```python
from build123d import *

# Parameters (mm, degrees)
BOSS_EXTRUDE1_DEPTH       = 35
BOSS_EXTRUDE3_DEPTH       = 1.5
SKETCH5_W                 = 1
SKETCH5_H                 = 1
BOSS_EXTRUDE4_DEPTH       = 18.1
CUT_EXTRUDE2_DEPTH        = 18.1
SKETCH9_W                 = 1
SKETCH9_H                 = 0.5
BOSS_EXTRUDE5_DEPTH       = 0.5
CUT_EXTRUDE3_REACH        = 41.512
SKETCH10_R                = 0.125
SKETCH11_R                = 2.5
BOSS_EXTRUDE6_DEPTH       = 1.5
SKETCH23_R                = 0.5
CUT_EXTRUDE12_DEPTH       = 1.5
SKETCH26_W                = 6.749879612
SKETCH26_H                = 8.598416767
SKETCH26_W_2              = 5.749879612
SKETCH26_H_2              = 7.598416767
BOSS_EXTRUDE16_DEPTH      = 2.05
BOSS_EXTRUDE23_REACH      = 41.419
BOSS_EXTRUDE23_END_RADIUS = 2.5
SKETCH27_W                = 0.594319842
SKETCH27_H                = 0.457567035
SKETCH27_R                = 0.154135996
SKETCH28_W                = 6.749879612
SKETCH28_H                = 8.598416767
BOSS_EXTRUDE24_DEPTH      = 0.5
SKETCH29_R                = 0.154135996
CUT_EXTRUDE13_DEPTH       = 2.5
SKETCH30_R                = 1.735676045
CUT_EXTRUDE14_DEPTH       = 0.5


with BuildPart() as part:
    # Sketch1 → Boss-Extrude1 (new body)
    with BuildSketch(Plane.XY):
        with BuildLine():
            Line((10.3, 6.55), (10.3, -6.55))
            ThreePointArc((10.3, -6.55), (9.567766953, -8.317766953), (7.8, -9.05))
            Line((7.8, -9.05), (-7.8, -9.05))
            Line((-7.8, -9.05), (-7.8, 9.05))
            Line((-7.8, 9.05), (7.8, 9.05))
            ThreePointArc((7.8, 9.05), (9.567766953, 8.317766953), (10.3, 6.55))
        make_face()
        with BuildLine():
            Line((-6.3, 7.55), (7.8, 7.55))
            ThreePointArc((7.8, 7.55), (8.507106781, 7.257106781), (8.8, 6.55))
            Line((8.8, 6.55), (8.8, -6.55))
            ThreePointArc((8.8, -6.55), (8.507106781, -7.257106781), (7.8, -7.55))
            Line((7.8, -7.55), (-6.3, -7.55))
            Line((-6.3, -7.55), (-6.3, 7.55))
        make_face(mode=Mode.SUBTRACT)
    extrude(amount=BOSS_EXTRUDE1_DEPTH)

    # Sketch4 → Boss-Extrude3 (add)
    with BuildSketch(Plane(origin=(0, 0, 0), x_dir=(-1, 0, 0), z_dir=(0, 0, -1))):
        with BuildLine():
            Line((7.8, -9.05), (7.8, 9.05))
            Line((7.8, 9.05), (-7.8, 9.05))
            ThreePointArc((-7.8, 9.05), (-9.567766953, 8.317766953), (-10.3, 6.55))
            Line((-10.3, 6.55), (-10.3, -6.55))
            ThreePointArc((-10.3, -6.55), (-9.567766953, -8.317766953), (-7.8, -9.05))
            Line((-7.8, -9.05), (7.8, -9.05))
        make_face()
    extrude(amount=-BOSS_EXTRUDE3_DEPTH)

    # Sketch5 → Boss-Extrude4 (add)
    with BuildSketch(Plane.XZ.offset(9.05)):
        with Locations((-8.3, 15)):
            Rectangle(SKETCH5_W, SKETCH5_H)
        with Locations((-8.3, 30)):
            Rectangle(SKETCH5_W, SKETCH5_H)
    extrude(amount=-BOSS_EXTRUDE4_DEPTH)

    # Sketch8 → Cut-Extrude2 (cut)
    with BuildSketch(Plane.ZY.offset(7.8)):
        with BuildLine():
            Line((0, -6.55), (0, -9.05))
            Line((0, -9.05), (2.5, -9.05))
            ThreePointArc((2.5, -9.05), (0.732233047, -8.317766953), (0, -6.55))
        make_face()
    extrude(amount=-CUT_EXTRUDE2_DEPTH, mode=Mode.SUBTRACT)

    # Sketch9 → Boss-Extrude5 (add)
    with BuildSketch(Plane.XY.offset(35)):
        with Locations((-5.5, -8.8)):
            Rectangle(SKETCH9_W, SKETCH9_H)
        with Locations((5.5, -8.8)):
            Rectangle(SKETCH9_W, SKETCH9_H)
    extrude(amount=BOSS_EXTRUDE5_DEPTH)

    # Cut-Extrude3: up to this face of the body (flat: up to its plane)
    cut_extrude3_end = Plane(part.part.faces().sort_by_distance((-6, -8.8, 35.25))[0])
    # Sketch10 → Cut-Extrude3 (cut, up to the picked face)
    with BuildSketch(Plane(origin=(6, 0, 0), x_dir=(0, 0, -1), z_dir=(1, 0, 0)), mode=Mode.PRIVATE) as cut_extrude3_sk1:
        with Locations((-35.25, -8.8)):
            Circle(SKETCH10_R)
    cut_extrude3_tool1 = split(extrude(cut_extrude3_sk1.sketch, amount=-CUT_EXTRUDE3_REACH, mode=Mode.PRIVATE), bisect_by=cut_extrude3_end, keep=Keep.BOTH, mode=Mode.PRIVATE)
    add(cut_extrude3_tool1.solids().sort_by(Axis((6, -8.8, 35.25), (-1, 0, 0)))[0], mode=Mode.SUBTRACT)

    # Sketch11 → Boss-Extrude6 (add)
    with BuildSketch(Plane.XY.offset(1.5)):
        with Locations(Location((0, 0, 0), (0, 0, 180))):
            Circle(SKETCH11_R)
    extrude(amount=BOSS_EXTRUDE6_DEPTH)

    # Sketch23 → Cut-Extrude12 (cut)
    with BuildSketch(Plane.ZY.offset(7.8)):
        with Locations(Location((6.47352849, -4.947355043, 0), (0, 0, 270))):
            Circle(SKETCH23_R)
    extrude(amount=-CUT_EXTRUDE12_DEPTH, mode=Mode.SUBTRACT)

    # Sketch26 → Boss-Extrude16 (add)
    with BuildSketch(Plane(origin=(-6.3, 0, 0), x_dir=(0, 0, -1), z_dir=(1, 0, 0))):
        with Locations((-4.874939806, -3.250791617)):
            Rectangle(SKETCH26_W, SKETCH26_H)
        with Locations((-4.874939806, -3.250791617)):
            Rectangle(SKETCH26_W_2, SKETCH26_H_2, mode=Mode.SUBTRACT)
    extrude(amount=BOSS_EXTRUDE16_DEPTH)

    # Boss-Extrude23: up to this cylinder (the profile starts outside it)
    boss_extrude23_end = Plane(origin=(0, 0, 2.254205), z_dir=(0, 0, -1)) * Cylinder(BOSS_EXTRUDE23_END_RADIUS, 88.838, mode=Mode.PRIVATE)
    # Sketch27 → Boss-Extrude23 (add, up to the surface)
    with BuildSketch(Plane(origin=(-4.25, 0, 0), x_dir=(0, 0, -1), z_dir=(1, 0, 0)), mode=Mode.PRIVATE) as boss_extrude23_sk1:
        with Locations((-2.25420487, 0.344193495)):
            Rectangle(SKETCH27_W, SKETCH27_H)
        with Locations(Location((-2.239067338, 0.317165037, 0), (0, 0, 270))):
            Circle(SKETCH27_R, mode=Mode.SUBTRACT)
    boss_extrude23_tool1 = extrude(boss_extrude23_sk1.sketch, amount=BOSS_EXTRUDE23_REACH, mode=Mode.PRIVATE) - boss_extrude23_end
    add(boss_extrude23_tool1.solids().sort_by_distance((-4.25, 0.565476, 2.254205))[0])

    # Sketch28 → Boss-Extrude24 (add)
    with BuildSketch(Plane(origin=(-4.25, 0, 0), x_dir=(0, 0, -1), z_dir=(1, 0, 0))):
        with Locations((-4.874939806, -3.250791617)):
            Rectangle(SKETCH28_W, SKETCH28_H)
    extrude(amount=BOSS_EXTRUDE24_DEPTH)

    # Sketch29 → Cut-Extrude13 (cut)
    with BuildSketch(Plane.ZY.offset(4.25)):
        with Locations((2.239067338, 0.317165037)):
            Circle(SKETCH29_R)
    extrude(amount=-CUT_EXTRUDE13_DEPTH, mode=Mode.SUBTRACT)

    # Sketch30 → Cut-Extrude14 (cut)
    with BuildSketch(Plane.XY.offset(3)):
        Circle(SKETCH30_R)
    extrude(amount=-CUT_EXTRUDE14_DEPTH, mode=Mode.SUBTRACT)


solid = part.part
```
Model file for the job. Use its own axes, mm. A direction names the side the tool comes from. Give positions to 0.01 mm unless a question says otherwise; leave off trailing zeros. Order: outer loops, then holes, each group sorted by start corner. A loop starts at its lowest first (then second) coordinate and runs counter-clockwise, first axis right, second up.
1) Mould opens along X. For faces 4 (the flat face through (-8, 0, 29.5)), 5 (the flat face through (-7.8, 0, 22)), 6 (the flat face through (-5, -3, 7.75)) say: +X half, -X half, draft (parallel to the pull), parting line (faces both ways), or undercut.
2) Wall check: probe 1 along Y at (x, z) = (0, 2.6); probe 2 along Y at (x, z) = (-1.5, 19.5); probe 3 along X at (y, z) = (1.5, 12). Give the ranges that are in metal, low to high.
3) Saw through at A-A, the plane z = 19.5. Write the cut outline in (x, y).
4) Saw through at C-C, the plane x = -0.75. Write the cut outline in (y, z), then the cut area to 3 significant figures.
5) Saw through at B-B, the plane y = 3.75. Write the cut outline in (x, z).
6) Pin check, flat tips, straight feed: pin 1 (4.5 mm diameter, centred on x = 0, y = 0, fed in from +Z); pin 2 (3 mm diameter, centred on x = 7.5, y = 2.5, fed in from +Z); pin 3 (2 mm diameter, centred on x = 4.5, y = -3, fed in from +Z); pin 4 (4 mm diameter, centred on y = -2.5, z = 13, fed in from -X). Stop position of each tip, or through.
7) 3-axis set-ups, long thin cutter, end or side, ignore diameter. For faces 1 (the flat face through (-1, -2, 3)), 2 (the flat face through (-8, 0, 14.5)), 3 (the flat face through (-8, 0, 15.5)): which of +Z, -Z, +X, -X, +Y, -Y reach the whole face in a straight line?
Computed:
1. face 4: draft
1. face 5: -X half
1. face 6: undercut
2. probe 1: y = -9.05 to -7.55, -2.5 to -1.74, 1.74 to 2.5, 7.55 to 9.05
2. probe 2: y = -9.05 to -7.55, 7.55 to 9.05
2. probe 3: x = -7.8 to -6.3, 8.8 to 10.3
3. outline: (-7.8, -9.05) - (7.8, -9.05) arc R2.5 ccw to (10.3, -6.55) - (10.3, 6.55) arc R2.5 ccw to (7.8, 9.05) - (-7.8, 9.05) - close; hole (-6.3, -7.55) - (7.8, -7.55) arc R1 ccw to (8.8, -6.55) - (8.8, 6.55) arc R1 ccw to (7.8, 7.55) - (-6.3, 7.55) - close
4. outline: (-9.05, 2.5) arc R2.5 ccw to (-6.55, 0) - (9.05, 0) - (9.05, 35) - (7.55, 35) - (7.55, 1.5) - (2.38, 1.5) - (2.38, 3) - (1.57, 3) - (1.57, 2.5) - (-1.57, 2.5) - (-1.57, 3) - (-2.38, 3) - (-2.38, 1.5) - (-7.55, 1.5) - (-7.55, 35) - (-9.05, 35) - close
4. area: 132 mm2
5. outline: (-8.8, 14.5) - (-7.8, 14.5) - (-7.8, 0) - (10.3, 0) - (10.3, 35) - (8.8, 35) - (8.8, 1.5) - (-6.3, 1.5) - (-6.3, 35) - (-7.8, 35) - (-7.8, 30.5) - (-8.8, 30.5) - (-8.8, 29.5) - (-7.8, 29.5) - (-7.8, 15.5) - (-8.8, 15.5) - close
6. pin 1: stops at z = 3
6. pin 2: stops at z = 35
6. pin 3: stops at z = 1.5
6. pin 4: stops at x = -8.8
7. face 1: +Z
7. face 2: -Z, -X, +Y, -Y
7. face 3: -X, +Y, -Y
